```python
from build123d import *

# Parameters (mm, degrees)
SKETCH_1_R          = 5
EXTRUDE_1_DEPTH     = 115
SKETCH_2_R          = 1
CUT_EXTRUDE_1_DEPTH = 10
SKETCH_4_R          = 1
CUT_EXTRUDE_2_DEPTH = 10


with BuildPart() as part:
    # Эскиз1 → Вытянуть1 (new body)
    with BuildSketch(Plane.XY):
        Circle(SKETCH_1_R)
    extrude(amount=EXTRUDE_1_DEPTH)

    # Эскиз2 → Вырез-Вытянуть1 (cut, symmetric)
    with BuildSketch(Plane(origin=(0, 0, 0), x_dir=(1, 0, 0), z_dir=(0, 1, 0))):
        with Locations(Location((0, -7.801268192, 0), (0, 0, 270))):
            Circle(SKETCH_2_R)
    extrude(amount=CUT_EXTRUDE_1_DEPTH, both=True, mode=Mode.SUBTRACT)

    # Эскиз4 → Вырез-Вытянуть2 (cut, symmetric)
    with BuildSketch(Plane(origin=(0, 0, 0), x_dir=(1, 0, 0), z_dir=(0, 1, 0))):
        with Locations(Location((0, -107.898465976, 0), (0, 0, 270))):
            Circle(SKETCH_4_R)
    extrude(amount=CUT_EXTRUDE_2_DEPTH, both=True, mode=Mode.SUBTRACT)


solid = part.part
```
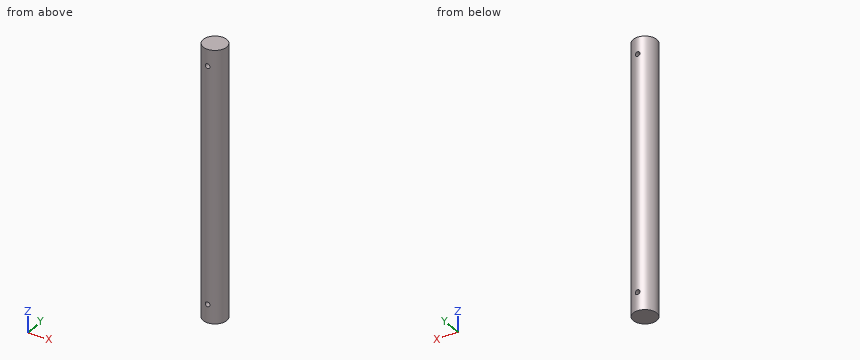
Design review of the part built by this model. Coordinates are the model's own, in mm. Give positions to 0.01 mm unless a question says otherwise; leave off trailing zeros. Loops run counter-clockwise (first coordinate to the right, second up) from the corner with the lowest first, then second, coordinate; pieces in that order, holes last. Notation, with made-up numbers: (54.5, 51.25) -> (95.5, 51.25) arc R20 cw to (95.5, 88.25) -> close; hole circle Ø11 at (-40, 23). An arc over 180 degrees is marked (long way). Write each question's results on one line, items separated by ' | '.
Q1. Take a section at D-D, the plane x = -3.75. Write out the cut boundary in (y, z).
Reply:
outline: (-3.31, 0) -> (3.31, 0) -> (3.31, 115) -> (-3.31, 115) -> close
Q2. For pin 1 Ø1.5 at (x, z) = (-3, 94.5) entering from -Y; pin 2 Ø1 at (y, z) = (2.5, 34.5) entering from -X; pin 3 Ø2 at (x, z) = (1.5, 43) entering from +Y; pin 4 Ø1 at (x, y) = (-0.5, 2.5) entering from -Z, all flat-tipped, find the tip position at first contact; note any pin that passes through.
Reply:
pin 1: stops at y = -4.47 | pin 2: stops at x = -4.58 | pin 3: stops at y = 4.97 | pin 4: stops at z = 0
Q3. Take a section at B-B, the plane z = 89. Write out the cut boundary in (x, y), plus the area to 3 significant figures.
Reply:
outline: circle Ø10 at (0, 0) | area: 78.5 mm²
Q4. Take a section at A-A, the plane y = 4. Write out the cut boundary in (x, z).
Reply:
outline: (-3, 0) -> (3, 0) -> (3, 115) -> (-3, 115) -> close; hole circle Ø2 at (0, 7.8); hole circle Ø2 at (0, 107.9)
Q5. Wall thickness on L1, parallel to Z at x = 0, y = -1; L2, parallel to Z at x = 0.75, y = -1.5; L3, parallel to X at y = -4.5, z = 8.5: over which ranges is each line inside the solid? List them lowest first.
Reply:
L1: z = 0 to 6.8, 8.8 to 106.9, 108.9 to 115 | L2: z = 0 to 7.14, 8.46 to 107.24, 108.56 to 115 | L3: x = -2.18 to -0.72, 0.72 to 2.18
Q6. Take a section at C-C, the plane y = -1.5. Write out the cut boundary in (x, z), plus the area to 3 significant figures.
Reply:
outline: (-4.77, 0) -> (4.77, 0) -> (4.77, 115) -> (-4.77, 115) -> close; hole circle Ø2 at (0, 7.8); hole circle Ø2 at (0, 107.9) | area: 1,090 mm²
